Part model, mm, in its own coordinate system. A direction names the side the tool comes from. Round coordinates to 2 decimals unless told otherwise and drop trailing zeros. Write each loop counter-clockwise with the first axis right and the second up, starting at its lowest first coordinate (ties: lowest second). Pieces come first, ordered by that corner, then holes. Notation, with made-up numbers: M 41,-19.75 L 80,-19.75 A14 ccw 80,-4.75 Z; hole C 57.25,14.5 d5. An arc over 180 degrees is marked long. One line per question, with ' | ' between items. Start each with the question number.
1) Wall check: probe 1 along X at (y, z) = (2.1, 2.75); probe 2 along X at (y, z) = (-0.55, 3.5); probe 3 along Z at (x, y) = (10.25, -0.9). Give the ranges that are in metal, low to high. Write a range as [from, to].
2) Tool access for faces 1 (the face through (-6.55, 2, 4)), 2 (the face through (-4, 2, -1.65)), 3 (the face through (-9.85, 2, 4)): list every direction of +Z, -Z, +X, -X, +Y, -Y with a clear straight run to the whole face (end or side of a thin tool).
3) Saw through at A-A (y = -0.3). List the corners of the cut face in (x, z), plus the area to 3 significant figures.
4) Mould opens along Z. For faces 4 (the face through (0, 1, 6)), 5 (the face through (-5.85, 2, 4)), 6 (the face through (-8, 2, -1.65)) say: pulls with the +Z half, pulls with the -Z half, needs draft (parallel to the pull), parting line crosses it, or undercut.
5) Saw through at D-D (y = 1.85). List the corners of the cut face in (x, z).
6) Drop flat-ended pins along their axis: pin 1 Ø1.4 at (y, z) = (-1, 4.5) entering from +X; pin 2 Ø4 at (x, z) = (-2.5, 2) entering from -Y; pin 3 Ø0.5 at (x, y) = (-9.5, -1) entering from +Z; pin 4 Ø0.6 at (x, z) = (-11, -3.5) entering from +Y. Give the stop position or say it passes through.
```python
from build123d import *

# Parameters (mm, degrees)
SKETCH1_W           = 25
SKETCH1_H           = 12
BOSS_EXTRUDE1_DEPTH = 1.6
SKETCH2_W           = 3.3
SKETCH2_H           = 3.3
SKETCH2_W_2         = 4.3
SKETCH2_H_2         = 6.6
BOSS_EXTRUDE2_DEPTH = 0.8
SKETCH3_W           = 2
SKETCH3_H           = 3
SKETCH3_W_2         = 5
SKETCH3_H_2         = 1.5
SKETCH3_W_3         = 2.5
SKETCH3_H_3         = 1.1
CUT_EXTRUDE1_DEPTH  = 0.01
SKETCH4_W           = 8.300946921
SKETCH4_H           = 3.688339109
SKETCH4_W_2         = 3.248116331
SKETCH4_H_2         = 9.777349986
SKETCH4_W_3         = 2.1
SKETCH4_H_3         = 2.1
SKETCH4_W_4         = 7.351587475
SKETCH4_H_4         = 2.509074224
BOSS_EXTRUDE3_DEPTH = 1.7


with BuildPart() as part:
    # Sketch1 → Boss-Extrude1 (new body)
    with BuildSketch(Plane(origin=(0, 0, 0), x_dir=(1, 0, 0), z_dir=(0, 1, 0))):
        Rectangle(SKETCH1_W, SKETCH1_H)
    extrude(amount=BOSS_EXTRUDE1_DEPTH)

    # Sketch2 → Boss-Extrude2 (add)
    with BuildSketch(Plane(origin=(0, 1.6, 0), x_dir=(1, 0, 0), z_dir=(0, 1, 0))):
        with Locations((-4.2, 4)):
            Rectangle(SKETCH2_W, SKETCH2_H)
        with Locations((-8.2, -4)):
            Rectangle(SKETCH2_W, SKETCH2_H)
        with Locations((-8.2, 4)):
            Rectangle(SKETCH2_W, SKETCH2_H)
        with Locations((-8.2, 0)):
            Rectangle(SKETCH2_W, SKETCH2_H)
        with Locations((-4.2, 0)):
            Rectangle(SKETCH2_W, SKETCH2_H)
        with Locations((-4.2, -4)):
            Rectangle(SKETCH2_W, SKETCH2_H)
        with Locations((4.95, 0)):
            Rectangle(SKETCH2_W_2, SKETCH2_H_2)
    extrude(amount=BOSS_EXTRUDE2_DEPTH)

    # Sketch3 → Cut-Extrude1 (cut)
    with BuildSketch(Plane(origin=(0, 1.6, 0), x_dir=(1, 0, 0), z_dir=(0, 1, 0))):
        with Locations((-11.25, 4.3)):
            Rectangle(SKETCH3_W, SKETCH3_H)
        with Locations((9.8, -4.45)):
            Rectangle(SKETCH3_W_2, SKETCH3_H_2)
        with Locations((-11.25, 0.3)):
            Rectangle(SKETCH3_W, SKETCH3_H)
        with Locations((-11.25, -3.7)):
            Rectangle(SKETCH3_W, SKETCH3_H)
        with Locations((9.8, 5.05)):
            Rectangle(SKETCH3_W_2, SKETCH3_H_2)
        with Locations((11.05, -2.15)):
            Rectangle(SKETCH3_W_3, SKETCH3_H_3)
        with Locations((11.05, -0.55)):
            Rectangle(SKETCH3_W_3, SKETCH3_H_3)
    extrude(amount=-CUT_EXTRUDE1_DEPTH, mode=Mode.SUBTRACT)

    # Sketch4 → Boss-Extrude3 (add)
    with BuildSketch(Plane.XZ):
        with Locations((7.251224506, -2.408711255)):
            Rectangle(SKETCH4_W, SKETCH4_H)
        with Locations((-9.853821619, 0)):
            Rectangle(SKETCH4_W_2, SKETCH4_H_2)
        with Locations((-4.089790985, 4.1)):
            Rectangle(SKETCH4_W_3, SKETCH4_H_3)
        with Locations((-4.089790985, 0)):
            Rectangle(SKETCH4_W_3, SKETCH4_H_3)
        with Locations((-4.089790985, -4.1)):
            Rectangle(SKETCH4_W_3, SKETCH4_H_3)
        with Locations((7.464495816, 4.579060458)):
            Rectangle(SKETCH4_W_4, SKETCH4_H_4)
    extrude(amount=BOSS_EXTRUDE3_DEPTH)


solid = part.part
```
Answer key:
1) probe 1: x = [-9.85, -6.55], [-5.85, -2.55], [2.8, 7.1] | probe 2: x = [-11.48, -8.23], [-5.14, -3.04], [3.79, 11.14] | probe 3: z = [-4.25, -0.56], [3.32, 5.83]
2) face 1: +Z, -Z, +Y | face 2: -X, +Y | face 3: +Z, -Z, -X, +Y
3) outline: M -11.48,-4.89 L -8.23,-4.89 L -8.23,4.89 L -11.48,4.89 Z; M -5.14,-5.15 L -3.04,-5.15 L -3.04,-3.05 L -5.14,-3.05 Z; M -5.14,-1.05 L -3.04,-1.05 L -3.04,1.05 L -5.14,1.05 Z; M -5.14,3.05 L -3.04,3.05 L -3.04,5.15 L -5.14,5.15 Z; M 3.1,-4.25 L 11.4,-4.25 L 11.4,-0.56 L 3.1,-0.56 Z; M 3.79,3.32 L 11.14,3.32 L 11.14,5.83 L 3.79,5.83 Z | area: 94.1 mm2
4) face 4: pulls with the +Z half | face 5: needs draft | face 6: undercut
5) outline: M -9.85,-5.65 L -6.55,-5.65 L -6.55,-2.35 L -9.85,-2.35 Z; M -9.85,-1.65 L -6.55,-1.65 L -6.55,1.65 L -9.85,1.65 Z; M -9.85,2.35 L -6.55,2.35 L -6.55,5.65 L -9.85,5.65 Z; M -5.85,-5.65 L -2.55,-5.65 L -2.55,-2.35 L -5.85,-2.35 Z; M -5.85,-1.65 L -2.55,-1.65 L -2.55,1.65 L -5.85,1.65 Z; M -5.85,2.35 L -2.55,2.35 L -2.55,5.65 L -5.85,5.65 Z; M 2.8,-3.3 L 7.1,-3.3 L 7.1,3.3 L 2.8,3.3 Z
6) pin 1: stops at x = 11.14 | pin 2: stops at y = -1.7 | pin 3: stops at z = 4.89 | pin 4: stops at y = 1.59
